Source: CAD feature listing. Evaluate the final solid. Frame: model axes, mm. Round coordinates to 2 decimals unless told otherwise and drop trailing zeros. Order: outer loops, then holes, each group sorted by start corner. A loop starts at its lowest first (then second) coordinate and runs counter-clockwise, first axis right, second up. Notation, with made-up numbers: (-31.75, 60.5) -> (-0.75, 60.5) arc R22 ccw to (-0.75, 97.5) -> close; hole circle Ø11 at (60.5, 88). An arc over 180 degrees is marked (long way). Answer as CSV lines item,"result".
from build123d import *

# Parameters (mm, degrees)
BOSS_EXTRUDE1_DEPTH = 6
CUT_EXTRUDE1_DEPTH  = 10


with BuildPart() as part:
    # Sketch1 → Boss-Extrude1 (new body)
    with BuildSketch(Plane(origin=(0, 0, 0), x_dir=(1, 0, 0), z_dir=(0, 1, 0))):
        Polygon((-160.386748432, 60.5), (-145.386748432, 60.5), (-145.386748432, -9.5), (-160.386748432, -9.5), (-160.386748432, -15.5), (-175.386748432, -15.5), (-175.386748432, -9.5), (-215.386748432, -9.5), (-215.386748432, -15.5), (-230.386748432, -15.5), (-230.386748432, -9.5), (-280.386748432, -9.5), (-280.386748432, -15.5), (-295.386748432, -15.5), (-295.386748432, -9.5), (-335.386748432, -9.5), (-335.386748432, -15.5), (-350.386748432, -15.5), (-350.386748432, -9.5), (-365.386748432, -9.5), (-365.386748432, 60.5), (-350.386748432, 60.5), (-350.386748432, 66.5), (-335.386748432, 66.5), (-335.386748432, 60.5), (-295.386748432, 60.5), (-295.386748432, 66.5), (-280.386748432, 66.5), (-280.386748432, 60.5), (-230.386748432, 60.5), (-230.386748432, 66.5), (-215.386748432, 66.5), (-215.386748432, 60.5), (-175.386748432, 60.5), (-175.386748432, 66.5), (-160.386748432, 66.5), align=None)
    extrude(amount=BOSS_EXTRUDE1_DEPTH)

    # Sketch2 → Cut-Extrude1 (cut)
    with BuildSketch(Plane.XZ):
        with BuildLine():
            Line((-350.386748432, -7), (-335.386748432, -7))
            ThreePointArc((-335.386748432, -7), (-327.886748432, -14.5), (-335.386748432, -22))
            Line((-335.386748432, -22), (-350.386748432, -22))
            ThreePointArc((-350.386748432, -22), (-357.886748432, -14.5), (-350.386748432, -7))
        make_face()
        with BuildLine():
            Line((-175.386748432, -22), (-160.386748432, -22))
            ThreePointArc((-160.386748432, -22), (-152.886748432, -14.5), (-160.386748432, -7))
            Line((-160.386748432, -7), (-175.386748432, -7))
            ThreePointArc((-175.386748432, -7), (-182.886748432, -14.5), (-175.386748432, -22))
        make_face()
    extrude(amount=-CUT_EXTRUDE1_DEPTH, mode=Mode.SUBTRACT)


solid = part.part
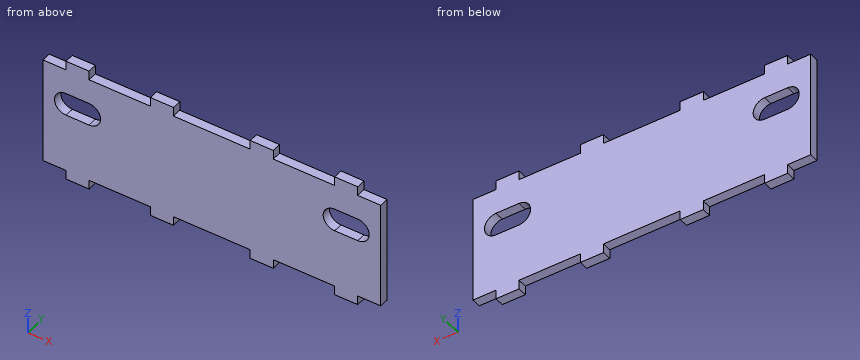
1. Section query C-C on y = 3.1. Give the number of separate pieces and of enclosed holes in the cut face, and give its area (3 significant figures).
Results below:
separate pieces,"1"
enclosed holes,"2"
area,"15,300 mm2"
2. Pin query (flat end, axial travel): pin 1 (3 mm diameter, centred on y = 4.5, z = 12.5, fed in from -X); pin 2 (3 mm diameter, centred on x = -153.5, y = 3, fed in from -Z); pin 3 (2 mm diameter, centred on x = -202, y = 4, fed in from +Z). Return the tip coordinate at first contact, or that it passes through.
Results below:
pin 1,"x = -350.39"
pin 2,"z = -60.5"
pin 3,"z = 9.5"
3. Section query B-B on x = -262. Return loops of the section in (y, z), and give its area (3 significant figures).
Results below:
outline,"(0, -60.5) -> (6, -60.5) -> (6, 9.5) -> (0, 9.5) -> close"
area,"420 mm2"
4. Section query A-A on z = -14.5. Return loops of the section in (x, y).
Results below:
outline,"(-365.39, 0) -> (-357.89, 0) -> (-357.89, 6) -> (-365.39, 6) -> close; (-327.89, 0) -> (-182.89, 0) -> (-182.89, 6) -> (-327.89, 6) -> close; (-152.89, 0) -> (-145.39, 0) -> (-145.39, 6) -> (-152.89, 6) -> close"
5. Line query: L1, parallel to X at y = 2.25, z = 10; L2, parallel to Z at x = -337.5, y = 0.3; L3, parallel to X at y = 4.85, z = -16. Output: solid intervals per line, ascending. Write a range as [from, to].
Results below:
L1,"[-350.39, -335.39], [-295.39, -280.39], [-230.39, -215.39], [-175.39, -160.39]"
L2,"[-66.5, -22], [-7, 15.5]"
L3,"[-365.39, -357.74], [-328.04, -182.74], [-153.04, -145.39]"
